Check sheet for the drawn part. Datum: minimum x, y, z corner. Units: mm. A direction names the side the tool comes from. Give positions to 0.01 mm unless a question says otherwise; leave off trailing zeros. Loops run counter-clockwise (first coordinate to the right, second up) from the corner with the lowest first, then second, coordinate; pieces in that order, holes last.
1. Cross-section at B-B, the plane x = 10. Record the cut outline in (y, z), plus the area to 3 significant figures.
2. Cross-section at C-C, the plane y = 12.5. Record the cut outline in (x, z), plus the area to 4 significant figures.
3. Go/stop test with flat-tipped pins: pin 1 Ø6 at (x, z) = (11, 6) entering from +Y; pin 2 Ø3 at (x, y) = (9, 17.5) entering from -Z; pin 3 Ø2.5 at (x, y) = (2.5, 16) entering from -Z. Record where each tip stops, or that it passes through.
4. Tool access check on the marked faces 1, 2 and 3. Record the directions out of +Z, -Z, +X, -X, +Y, -Y that give a thin tool (end or side, any length) a straight path to the whole face; none if there is none.
5. Cross-section at D-D, the plane z = 5.5. Record the cut outline in (x, y).
6. Material ranges on L1, parallel to Z at x = 10, y = 7.75; L2, parallel to X at y = 7.5, z = 7.5; L3, parallel to X at y = 14.75, z = 29.5, recorded low to high.
7. Release check for a two-part mould opening along Z. For the marked faces 4, 5 and 6 record: +Z half, -Z half, draft (parallel to the pull), parting line (faces both ways), or undercut.
8. Cross-section at A-A, the plane z = 10. Record the cut outline in (x, y), plus the area to 3 significant figures.
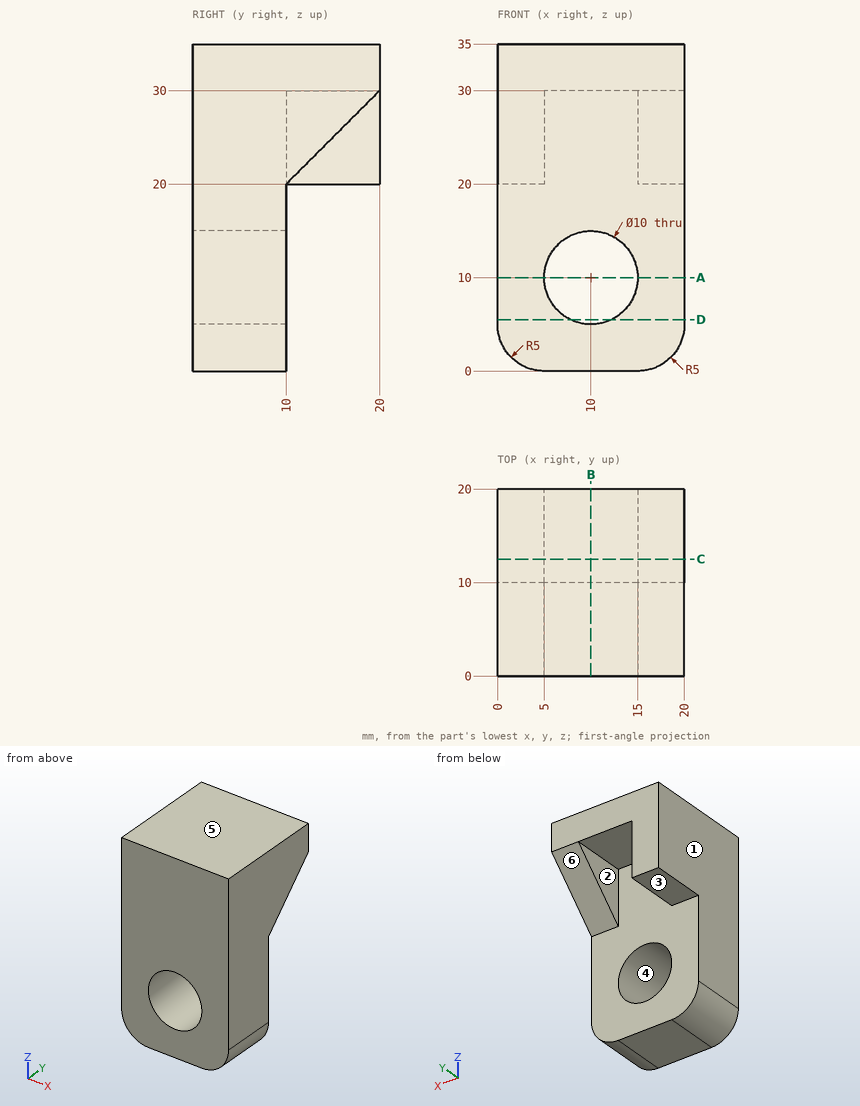
Result:
1. outline: (0, 0) - (10, 0) - (10, 5) - (0, 5) - close; (0, 15) - (10, 15) - (10, 30) - (20, 30) - (20, 35) - (0, 35) - close
1. area: 300 mm2
2. outline: (0, 20) - (5, 20) - (5, 30) - (15, 30) - (15, 22.5) - (20, 22.5) - (20, 35) - (0, 35) - close
2. area: 187.5 mm2
3. pin 1: stops at y = 10
3. pin 2: stops at z = 30
3. pin 3: stops at z = 20
4. face 1: +Z, -Z, -X, +Y, -Y
4. face 2: -Z, +Y
4. face 3: -Z, +X, -X, +Y
5. outline: (0, 0) - (7.82, 0) - (7.82, 10) - (0, 10) - close; (12.18, 0) - (20, 0) - (20, 10) - (12.18, 10) - close
6. L1: z = 0 to 5, 15 to 35
6. L2: x = 0 to 5.67, 14.33 to 20
6. L3: x = 0 to 5, 15 to 20
7. face 4: undercut
7. face 5: +Z half
7. face 6: -Z half
8. outline: (0, 0) - (5, 0) - (5, 10) - (0, 10) - close; (15, 0) - (20, 0) - (20, 10) - (15, 10) - close
8. area: 100 mm2
